The listing builds one solid part. Answer for the finished solid, in the listing's coordinates (mm). A direction names the side the tool comes from. Coordinates: 2 decimals unless noted, no trailing zeros. Write each loop counter-clockwise with the first axis right and the second up, starting at its lowest first coordinate (ties: lowest second). Pieces come first, ordered by that corner, then holes.
(1) Which of the six approach directions +Z, -Z, +X, -X, +Y, -Y give full straight-line access (tool end or side, diameter ignored) to faces 4 (the flat face through (-1, -38.1, 1)), 5 (the flat face through (-72.736, -1, -1)), 6 (the cylindrical face through (-0.725, 44.361, 8.087))?
(2) The part is cut by section A-A on y = 0. Determine the outline of the cut face in (x, z).
(3) Straight lines are drawn through the part: line 1 (Y direction, x = 53, z = -7); line 2 (Y direction, x = 38.5, z = -5); line 3 (X direction, y = 1.5, z = 21). For each, find the intervals that lie inside material, in ascending order.
(4) For a pull along X with two mould halves and no side action, classify faces 1 (the cylindrical face through (0.531, 0.711, 16.872)), 2 (the flat face through (72.736, -1, -1)), 3 (the flat face through (-1, 38.1, 1)) as +X half, -X half, draft (parallel to the pull), parting line (faces both ways), or undercut.
(5) The part is cut by section D-D on x = 0. Determine the outline of the cut face in (y, z).
(6) The part is cut by section B-B on z = 34.5. Determine the outline of the cut face in (x, y), plus the area to 3 significant figures.
(7) The part is cut by section C-C on z = 1.5. Determine the outline of the cut face in (x, y).
(8) Given P1, Ø3, axis at x = 1.5, y = 23.5, coming from the +Z side; P2, Ø8, axis at x = 34, z = -5.5, coming from the +Y side; P3, Ø1, axis at y = -39, z = 19, coming from the +X side, each flat-ended and moving along its own axis, determine where each tip first touches the part or whether it passes through.
from build123d import *

# Parameters (mm, degrees)
F0_W          = 145.4727351665
F0_H          = 82.0685699582
F1_DEPTH      = 38.1
F3_DEPTH      = 12.7
F3_DEPTH_BACK = 88.9
F4_DEPTH      = 88.901
F6_D          = 25.4


with BuildPart() as f1:
    # F0 (on Front) → F1 (new body, symmetric)
    with BuildSketch(Plane.XZ):
        Rectangle(F0_W, F0_H)
    extrude(amount=F1_DEPTH, both=True)

    # F2 (on face) → F3 (join, two sides)
    with BuildSketch(Plane.XZ.offset(38.1)) as f3_sk:
        with BuildLine():
            Line((-24.1679944094, 41.0342849791), (-32.9555145721, 41.0342849791))
            ThreePointArc((-32.9555145721, 41.0342849791), (0, 8.078770407), (32.9555145721, 41.0342849791))
            Line((32.9555145721, 41.0342849791), (24.1679944094, 41.0342849791))
            ThreePointArc((24.1679944094, 41.0342849791), (0, 16.8662905697), (-24.1679944094, 41.0342849791))
        make_face()
    extrude(amount=F3_DEPTH)
    extrude(f3_sk.sketch, amount=-F3_DEPTH_BACK)

    # F4 (cut, through all): a face of the model
    f4_faces = [f1.faces().sort_by_distance(p)[0] for p in [
        (0, -38.1, 30.7770695794),
    ]]
    extrude(f4_faces, amount=-F4_DEPTH, mode=Mode.SUBTRACT)

    # F6 (through all)
    with Locations(Plane.XY.offset(41.0342849791)):
        with Locations((-50.2582862973, 0), (52.3969344795, 0)):
            Hole(F6_D / 2)


solid = f1.part
Model answer:
1. face 4: -Z, -Y
1. face 5: +Z, -Z, -X, +Y, -Y
1. face 6: -Z, +Y
2. outline: (-72.74, -41.03) - (-62.96, -41.03) - (-62.96, 41.03) - (-72.74, 41.03) - close; (-37.56, -41.03) - (39.7, -41.03) - (39.7, 41.03) - (24.17, 41.03) arc R24.17 cw to (-24.17, 41.03) - (-37.56, 41.03) - close; (65.1, -41.03) - (72.74, -41.03) - (72.74, 41.03) - (65.1, 41.03) - close
3. line 1: y = -38.1 to -12.69, 12.69 to 38.1
3. line 2: y = -38.1 to 38.1
3. line 3: x = -72.74 to -62.87, -37.65 to -13.52, 13.52 to 39.79, 65.01 to 72.74
4. face 1: undercut
4. face 2: +X half
4. face 3: draft
5. outline: (-50.8, 8.08) - (-38.1, 8.08) - (-38.1, -41.03) - (38.1, -41.03) - (38.1, 8.08) - (50.8, 8.08) - (50.8, 16.87) - (-50.8, 16.87) - close
6. outline: (-72.74, -38.1) - (-32.3, -38.1) - (-32.3, -50.8) - (-23.27, -50.8) - (-23.27, 50.8) - (-32.3, 50.8) - (-32.3, 38.1) - (-72.74, 38.1) - close; (23.27, -50.8) - (32.3, -50.8) - (32.3, -38.1) - (72.74, -38.1) - (72.74, 38.1) - (32.3, 38.1) - (32.3, 50.8) - (23.27, 50.8) - close; hole circle Ø25.4 at (-50.26, 0); hole circle Ø25.4 at (52.4, 0)
6. area: 6,980 mm2
7. outline: (-72.74, -38.1) - (72.74, -38.1) - (72.74, 38.1) - (-72.74, 38.1) - close; hole circle Ø25.4 at (-50.26, 0); hole circle Ø25.4 at (52.4, 0)
8. P1: stops at z = 17.05
8. P2: stops at y = 38.1
8. P3: stops at x = 24.95
